```python
from build123d import *

# Parameters (mm, degrees)
F1_DEPTH = 27.94
F3_DEPTH = 25.146
F4_R     = 2.921
F6_DEPTH = 3.048
F5_R     = 2.921
F7_DEPTH = 3.048
F9_DEPTH = 5.08


with BuildPart() as f1:
    # F0 (on Front) → F1 (new body)
    with BuildSketch(Plane.XZ):
        with BuildLine():
            Line((0, 123.19), (-25.4, 123.19))
            Line((-25.4, 123.19), (-25.4, 0))
            Line((-25.4, 0), (-19.05, 0))
            ThreePointArc((-19.05, 0), (-5.579616, 5.579616), (0, 19.05))
            Line((0, 19.05), (0, 123.19))
        make_face()
    extrude(amount=F1_DEPTH)

    # F2 (on face) → F3 (cut)
    with BuildSketch(Plane.YZ):
        Polygon((-1.27, -9.116447), (-1.27, 19.05), (-26.67, 19.05), (-26.67, -8.348415), align=None)
        Polygon((-1.27, 19.05), (-1.27, 20.321167), (-1.27, 121.92), (-26.67, 121.92), (-26.67, 20.32), (-26.67, 19.05), align=None)
    extrude(amount=-F3_DEPTH, mode=Mode.SUBTRACT)

    # F4 (on face) → F6 (join)
    with BuildSketch(Plane(origin=(0, -26.67, 0), x_dir=(-1, 0, 0), z_dir=(0, 1, 0))):
        with Locations((12.7, 12.7)):
            Circle(F4_R)
    extrude(amount=F6_DEPTH)

    # F5 (on face) → F7 (join)
    with BuildSketch(Plane.XZ.offset(1.27)):
        with Locations((-12.7, 12.7)):
            Circle(F5_R)
    extrude(amount=F7_DEPTH)

    # F8 (on face) → F9 (cut)
    with BuildSketch(Plane(origin=(-25.4, 0, 0), x_dir=(0, -1, 0), z_dir=(-1, 0, 0))):
        Polygon((26.67, 23.318777), (1.27, 23.318777), (1.27, 0.254), (1.27, 0), (26.67, 0), (26.67, 0.254), align=None)
    extrude(amount=-F9_DEPTH, mode=Mode.SUBTRACT)


solid = f1.part
```
Input: part model. Units: mm. Frame: model coordinates. A direction names the side the tool comes from. Round coordinates to 2 decimals unless told otherwise and drop trailing zeros. Write each loop counter-clockwise with the first axis right and the second up, starting at its lowest first coordinate (ties: lowest second). Pieces come first, ordered by that corner, then holes. Notation, with made-up numbers: (86.5, 87.25) -> (140.5, 87.25) arc R5 ccw to (140.5, 94.25) -> close; hole circle Ø6 at (68, -34.75). An arc over 180 degrees is marked (long way). Answer as CSV lines item,"result".
1. Mould query, pull axis Y, two halves, no side actions, for faces 1 (the flat face through (-13, -27.94, 62)), 2 (the flat face through (-13, -4.318, 13)), 3 (the flat face through (-25.4, -14, 76)). Classes: +Y half, -Y half, draft (parallel to the pull), parting line (faces both ways), or undercut.
Geometry says:
face 1,"-Y half"
face 2,"undercut"
face 3,"draft"
2. Section C-C (x = -4.5). Return the cut outline in (y, z), plus the area to 3 significant figures.
Geometry says:
outline,"(-27.94, 6.75) -> (-26.67, 6.75) -> (-26.67, 121.92) -> (-1.27, 121.92) -> (-1.27, 6.75) -> (0, 6.75) -> (0, 123.19) -> (-27.94, 123.19) -> close"
area,"328 mm^2"
3. Contact query for flat-ended pins moving along their axis: P1, Ø4, axis at x = -17.5, y = -11.5, coming from the -Z side; P2, Ø1, axis at y = -3, z = 16.5, coming from the +X side (3 decimals); P3, Ø8, axis at x = -18, y = -6.5, coming from the -Z side. Output: stop coordinate, or through.
Geometry says:
P1,"stops at z = 121.92"
P2,"passes through"
P3,"stops at z = 10.52"
4. Reachability of faces 4 (the flat face through (-13, -14, 123.19)), 5 (the flat face through (0, -0.5, 70.9)), 6 (the cylindrical face through (-15.398, -25.167, 11.581)), 7 (the flat face through (-25.146, -14, 73)), 8 (the flat face through (-13, -23.622, 13)) from +Z, -Z, +X, -X, +Y, -Y: full face, straight path, thin tool, end or side. Return the list, or none.
Geometry says:
face 4,"+Z, +X, -X, +Y, -Y"
face 5,"+Z, -Z, +X, +Y, -Y"
face 6,"none"
face 7,"-Z, +X"
face 8,"-Z, +X, -X"
5. Section A-A (z = 12.7). Return the cut outline in (x, y).
Geometry says:
outline,"(-25.4, -27.94) -> (-1.09, -27.94) -> (-1.09, -26.67) -> (-9.78, -26.67) -> (-9.78, -23.62) -> (-15.62, -23.62) -> (-15.62, -26.67) -> (-25.4, -26.67) -> close; (-25.4, -1.27) -> (-15.62, -1.27) -> (-15.62, -4.32) -> (-9.78, -4.32) -> (-9.78, -1.27) -> (-1.09, -1.27) -> (-1.09, 0) -> (-25.4, 0) -> close"
6. Section D-D (y = -18.75). Return the cut outline in (x, z), plus the area to 3 significant figures.
Geometry says:
outline,"(-25.4, 23.32) -> (-25.15, 23.32) -> (-25.15, 121.92) -> (0, 121.92) -> (0, 123.19) -> (-25.4, 123.19) -> close"
area,"57.3 mm^2"
7. Ray query, L1, parallel to Y at x = -8.5, z = 108; L2, parallel to Z at x = -24, y = -3.75; L3, parallel to X at y = -12.5, z = 87. Return the intervals inside material, ascending. Write a range as [from, to].
Geometry says:
L1,"y = [-27.94, -26.67], [-1.27, 0]"
L2,"z = [121.92, 123.19]"
L3,"x = [-25.4, -25.15]"
8. Section B-B (z = 92). Return the cut outline in (x, y), plus the area to 3 significant figures.
Geometry says:
outline,"(-25.4, -27.94) -> (0, -27.94) -> (0, -26.67) -> (-25.15, -26.67) -> (-25.15, -1.27) -> (0, -1.27) -> (0, 0) -> (-25.4, 0) -> close"
area,"71.0 mm^2"
